The model under review builds one solid part; all positions refer to its coordinate system, in mm. Face numbers are marked on the shaded views. A direction names the side the tool comes from. Coordinates: 2 decimals unless noted, no trailing zeros. Use CSV: the item, a comma, the result in double quotes. Start each with the question number.
1. For L1, parallel to Y at x = 0, z = 10.5 (3 decimals); L2, parallel to X at y = 105, z = 224, list the stretches that pass through material, from the lowest coordinate up.
2. Tool access review of the marked faces 1 and 2: name each direction out of +Z, -Z, +X, -X, +Y, -Y from which nothing blocks a thin tool from reaching the whole face with its end or side.
3. Clearance check with flat-ended pins moving along their axes: P1, Ø12, axis at x = -1, y = 1.5, coming from the +Z side; P2, Ø8, axis at x = -21, y = 91.5, coming from the +Z side; P3, Ø1, axis at x = -11.5, y = 92, coming from the +Z side. State where each tip first meets the part, or that it passes through.
from build123d import *

# Parameters (mm, degrees)
SWEEP1_PROFILE_R     = 13.49375
CUT_SWEEP1_PROFILE_R = 9.525


with BuildPart() as part:
    # Sweep1: sweep along a curve in space
    with BuildLine() as sweep1_path:
        Line((0, 0, 0), (0, 0, -25.4))
        Line((0, 0, 0), (0, 0, 65.008326235))
        ThreePointArc((-5.864570369, 12.64082052, 138.960948382), (-1.478930869, 3.187769693, 102.635357248), (0, 0, 65.008326235))
        ThreePointArc((-11.705580718, 100.75868887, 220.409758136), (-12.308159492, 46.60541038, 190.353572184), (-5.864570369, 12.64082052, 138.960948382))
        Line((-10.149398836, 122.948822825, 226.479981937), (-11.705580718, 100.75868887, 220.409758136))
    # Sweep1 profile (on start of the path) → Sweep1 (sweep)
    with BuildSketch(Plane(origin=(-10.149398836, 122.948822825, 226.479981937), x_dir=(0, 0.26386051670744176, -0.9645608470816561), z_dir=(-0.06748988993383706, -0.9623616079186076, -0.2632589036690513))):
        Circle(SWEEP1_PROFILE_R)
    sweep(path=sweep1_path.line)

    # Cut-Sweep1: sweep along a curve in space
    with BuildLine() as cut_sweep1_path:
        Line((0, 0, 0), (0, 0, -25.4))
        Line((0, 0, 0), (0, 0, 65.008326235))
        ThreePointArc((-5.864570369, 12.64082052, 138.960948382), (-1.478930869, 3.187769693, 102.635357248), (0, 0, 65.008326235))
        ThreePointArc((-11.705580718, 100.75868887, 220.409758136), (-12.308159492, 46.60541038, 190.353572184), (-5.864570369, 12.64082052, 138.960948382))
        Line((-10.149398836, 122.948822825, 226.479981937), (-11.705580718, 100.75868887, 220.409758136))
    # Cut-Sweep1 profile (on start of the path) → Cut-Sweep1 (sweep, cut)
    with BuildSketch(Plane(origin=(-10.149398836, 122.948822825, 226.479981937), x_dir=(0, 0.26386051670744176, -0.9645608470816561), z_dir=(-0.06748988993383706, -0.9623616079186076, -0.2632589036690513))):
        Circle(CUT_SWEEP1_PROFILE_R)
    sweep(path=cut_sweep1_path.line, mode=Mode.SUBTRACT)


solid = part.part
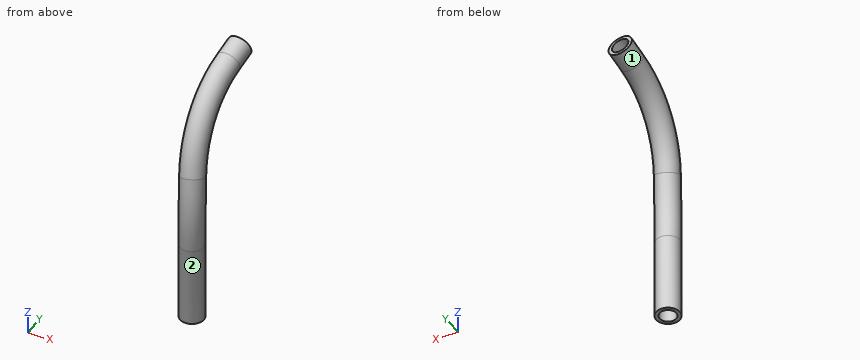
Computed:
1,L1,"y = -13.494 to -9.525, 9.525 to 13.494"
1,L2,"x = -24.68 to -20.62, -2.11 to 1.95"
2,face 1,"none"
2,face 2,"-Z"
3,P1,"stops at z = 158.22"
3,P2,"stops at z = 231.1"
3,P3,"stops at z = 232.05"
